Build history of the part. All positions in model axes, mm. A direction names the side the tool comes from. Coordinates: 2 decimals unless noted, no trailing zeros. Order: outer loops, then holes, each group sorted by start corner. A loop starts at its lowest first (then second) coordinate and runs counter-clockwise, first axis right, second up. Notation, with made-up numbers: M 34,21 L 77,21 A18 cw 77,35 Z; hole C -28,79.5 d3. An arc over 180 degrees is marked long. Use a Markdown table: item, result. Add a question column.
from build123d import *

# Parameters (mm, degrees)
SKETCH1_R           = 30
BOSS_EXTRUDE1_DEPTH = 6.35
SKETCH2_R           = 1.4224
CUT_EXTRUDE1_DEPTH  = 6.35


with BuildPart() as part:
    # Sketch1 → Boss-Extrude1 (new body)
    with BuildSketch(Plane(origin=(0, 0, 0), x_dir=(0, 0, -1), z_dir=(1, 0, 0))):
        Polygon((0, 0), (70, 0), (70, 49.756615014), (64.872483647, 54.884131367), (70, 60.011647719), (70, 70), (60.148635267, 70), (54.952625141, 64.803989874), (49.756615014, 70), (0, 70), align=None)
        with Locations((35, 35)):
            Circle(SKETCH1_R, mode=Mode.SUBTRACT)
    extrude(amount=BOSS_EXTRUDE1_DEPTH)

    # Sketch2 → Cut-Extrude1 (cut)
    with BuildSketch(Plane(origin=(6.35, 0, 0), x_dir=(0, 0, -1), z_dir=(1, 0, 0))):
        with Locations((8.707441752, 61.25)):
            Circle(SKETCH2_R)
        with Locations((8.707441752, 8.75)):
            Circle(SKETCH2_R)
        with Locations((61.292558248, 8.75)):
            Circle(SKETCH2_R)
    extrude(amount=-CUT_EXTRUDE1_DEPTH, mode=Mode.SUBTRACT)


solid = part.part
(1) Slice it at B-B on z = -35. Give the cut face in (x, y).
(2) Drill centre lines: line 1 along Y through (x, z) = (2.25, -35); line 2 along Z through (x, y) = (5.5, 59); line 3 along Y through (x, z) = (3.5, -66). Where is each one in solid material? Low to high. Write a range as from..to.
(3) Slice it at D-D on y = 8.75. Give the cut face in (x, z), and give its area (3 significant figures).
(4) Slice it at A-A on y = 17. Give the cut face in (x, z).
(5) Which spindle directions (+Z, -Z, +X, -X, +Y, -Y) get a long thin tool onto all of the face, cutting with end or side? Do faces 1 (the flat face through (3.131, 67.366, -52.391)), 2 (the flat face through (3, 70, -65)), 3 (the flat face through (3.13, 57.41, -67.4)). Say none if no direction does.
(6) Mould opens along Y. For faces 4 (the flat face through (3, 0, -35)), 5 (the flat face through (3, 25, -70)), 6 (the flat face through (3.131, 52.284, -67.472)) say: released by +Y, released by -Y, zero draft, split by the parting line, or undercut.
(7) Slice it at C-C on x = 4.75. Give the cut face in (y, z).
Solutions:
| question | item | result |
|---|---|---|
| 1 | outline | M 0,0 L 6.35,0 L 6.35,5 L 0,5 Z; M 0,65 L 6.35,65 L 6.35,70 L 0,70 Z |
| 2 | line 1 | 0..5, 65..70 |
| 2 | line 2 | -68.99..-53, -17..0 |
| 2 | line 3 | 0..53.76, 56.01..70 |
| 3 | outline | M 0,-70 L 6.35,-70 L 6.35,-62.71 L 0,-62.71 Z; M 0,-59.87 L 6.35,-59.87 L 6.35,-49.52 L 0,-49.52 Z; M 0,-20.48 L 6.35,-20.48 L 6.35,-10.13 L 0,-10.13 Z; M 0,-7.29 L 6.35,-7.29 L 6.35,0 L 0,0 Z |
| 3 | area | 224 mm² |
| 4 | outline | M 0,-70 L 6.35,-70 L 6.35,-59 L 0,-59 Z; M 0,-11 L 6.35,-11 L 6.35,0 L 0,0 Z |
| 5 | face 1 | +X, -X, +Y |
| 5 | face 2 | +Z, -Z, +X, -X, +Y |
| 5 | face 3 | -Z, +X, -X |
| 6 | face 4 | released by -Y |
| 6 | face 5 | zero draft |
| 6 | face 6 | undercut |
| 7 | outline | M 0,-70 L 49.76,-70 L 54.88,-64.87 L 60.01,-70 L 70,-70 L 70,-60.15 L 64.8,-54.95 L 70,-49.76 L 70,0 L 0,0 Z; hole C 35,-35 d60; hole C 8.75,-61.29 d2.84; hole C 8.75,-8.71 d2.84; hole C 61.25,-8.71 d2.84 |
